Check sheet for the drawn part. Datum: minimum x, y, z corner. Units: mm. Round coordinates to 2 decimals unless told otherwise and drop trailing zeros. Order: outer loops, then holes, each group sorted by start corner. A loop starts at its lowest first (then second) coordinate and runs counter-clockwise, first axis right, second up. Notation, with made-up numbers: (17.25, 66.5) -> (30.25, 66.5) arc R13 ccw to (30.25, 74.5) -> close; hole circle Ø6 at (0.5, 26.25). An arc over 180 degrees is marked (long way). Write item = value, one per line. Start each with the question number.
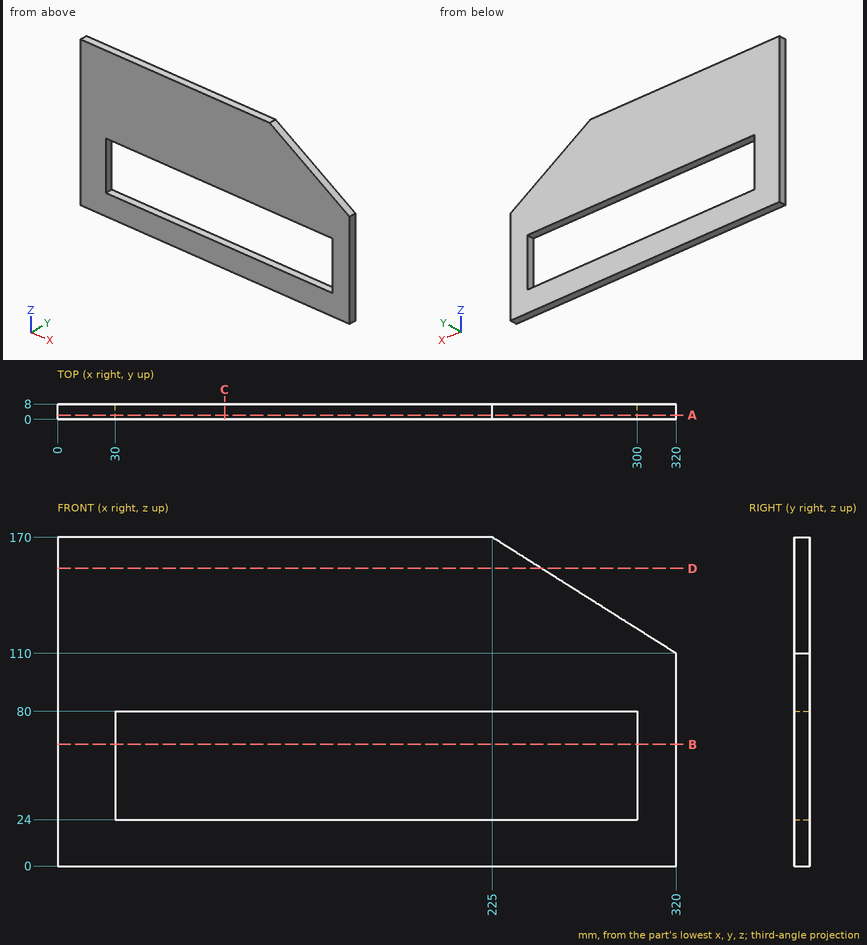
(1) Cross-section at C-C (x = 86.5). Enter the section's corners in (y, z), and give its area (3 significant figures).
(2) Cross-section at A-A (y = 2.25). Enter the section's corners in (x, z), and give its area (3 significant figures).
(3) Cross-section at D-D (z = 154). Enter the section's corners in (x, y).
(4) Cross-section at B-B (z = 63). Enter the section's corners in (x, y).
(5) Scan lines: line 1 along X through (y, z) = (7, 31); line 2 along Z through (x, y) = (146, 0.75); line 3 along Z through (x, y) = (251.5, 2.25). Record each from-to range of solid material in increasing order. Write a range as from..to.
Outcome:
q1.outline = (0, 0) -> (8, 0) -> (8, 24) -> (0, 24) -> close; (0, 80) -> (8, 80) -> (8, 170) -> (0, 170) -> close
q1.area = 912 mm^2
q2.outline = (0, 0) -> (320, 0) -> (320, 110) -> (225, 170) -> (0, 170) -> close; hole (30, 24) -> (300, 24) -> (300, 80) -> (30, 80) -> close
q2.area = 36,400 mm^2
q3.outline = (0, 0) -> (250.33, 0) -> (250.33, 8) -> (0, 8) -> close
q4.outline = (0, 0) -> (30, 0) -> (30, 8) -> (0, 8) -> close; (300, 0) -> (320, 0) -> (320, 8) -> (300, 8) -> close
q5.line_1 = 0..30, 300..320
q5.line_2 = 0..24, 80..170
q5.line_3 = 0..24, 80..153.26
